Read the model definition and answer for the solid it produces. Units are mm, in the model's axes. A direction names the side the tool comes from. Round coordinates to 2 decimals unless told otherwise and drop trailing zeros. Write each loop counter-clockwise with the first axis right and the second up, starting at its lowest first coordinate (ties: lowest second). Pieces come first, ordered by that corner, then holes. Notation, with made-up numbers: M 21,-13 L 79,-13 A5 cw 79,-7 Z; hole C -14.5,47 d2. An arc over 180 degrees is marked long. Use one line per item in the form item = value. Start each with the question number.
```python
from build123d import *

# Parameters (mm, degrees)
SKETCH1_W               = 101.6
SKETCH1_H               = 6.35
BOSS_EXTRUDE1_DEPTH     = 101.6
CUT_EXTRUDE1_DEPTH      = 144.824345992
SKETCH5_R               = 2.0828
CUT_EXTRUDE2_DEPTH      = 144.824345992
MIRROR2_COPY_1_SKETCH_R = 2.0828
MIRROR2_COPY_1_DEPTH    = 144.824345992


with BuildPart() as part:
    # Sketch1 → Boss-Extrude1 (new body)
    with BuildSketch(Plane(origin=(0, 0, 0), x_dir=(1, 0, 0), z_dir=(0, 1, 0))):
        with Locations((50.8, 3.175)):
            Rectangle(SKETCH1_W, SKETCH1_H)
    extrude(amount=BOSS_EXTRUDE1_DEPTH)

    # Sketch2 → Cut-Extrude1 (cut, through all)
    with BuildSketch(Plane(origin=(0, 0, -6.35), x_dir=(-1, 0, 0), z_dir=(0, 0, -1))):
        with BuildLine():
            Line((-88.9, 66.294), (-12.7, 66.294))
            ThreePointArc((-12.7, 66.294), (-9.906, 63.5), (-12.7, 60.706))
            Line((-12.7, 60.706), (-88.9, 60.706))
            ThreePointArc((-88.9, 60.706), (-91.694, 63.5), (-88.9, 66.294))
        make_face()
        with BuildLine():
            Line((-88.9, 40.894), (-12.7, 40.894))
            ThreePointArc((-12.7, 40.894), (-9.906, 38.1), (-12.7, 35.306))
            Line((-12.7, 35.306), (-88.9, 35.306))
            ThreePointArc((-88.9, 35.306), (-91.694, 38.1), (-88.9, 40.894))
        make_face()
    extrude(amount=-CUT_EXTRUDE1_DEPTH, mode=Mode.SUBTRACT)

    # Sketch5 → Cut-Extrude2 (cut, through all)
    with BuildSketch(Plane.XY):
        with Locations((19.431, 85.725)):
            Circle(SKETCH5_R)
        with Locations((38.481, 95.25)):
            Circle(SKETCH5_R)
        with Locations((38.481, 76.2)):
            Circle(SKETCH5_R)
        with Locations((57.531, 85.725)):
            Circle(SKETCH5_R)
    cut_extrude2 = extrude(amount=-CUT_EXTRUDE2_DEPTH, mode=Mode.SUBTRACT)

    # Mirror1: Cut-Extrude2 across plane
    add(cut_extrude2.mirror(Plane.ZX.offset(50.8)), mode=Mode.SUBTRACT)

    # Mirror2: Cut-Extrude2 across plane
    add(cut_extrude2.mirror(Plane(origin=(48.41875, 0, 0), x_dir=(0, 0, 1), z_dir=(1, 0, 0))), mode=Mode.SUBTRACT)

    # Mirror2 copy 1 sketch → Mirror2 copy 1 (cut, through all)
    with BuildSketch(Plane(origin=(96.8375, 101.6, 0), x_dir=(-1, 0, 0), z_dir=(0, 0, 1))):
        with Locations((19.431, 85.725)):
            Circle(MIRROR2_COPY_1_SKETCH_R)
        with Locations((38.481, 95.25)):
            Circle(MIRROR2_COPY_1_SKETCH_R)
        with Locations((38.481, 76.2)):
            Circle(MIRROR2_COPY_1_SKETCH_R)
        with Locations((57.531, 85.725)):
            Circle(MIRROR2_COPY_1_SKETCH_R)
    extrude(amount=-MIRROR2_COPY_1_DEPTH, mode=Mode.SUBTRACT)


solid = part.part
```
Q1. Find section A-A on y = 6.35. Write down the section's boundary in (x, z).
Q2. Straight lines are drawn through the part: line 1 (X direction, y = 6.35, z = -1.25); line 2 (Y direction, x = 53.5, z = -3); line 3 (X direction, y = 6, z = -1.5). For each, find the intervals that lie inside material, in ascending order. Write a range as [from, to].
Q3. Find section B-B on x = 62. Write down the section's boundary in (y, z).
Q4. For a pull along Y with two mould halves and no side action, classify faces 3 (the face through (50, 0, -3)), 4 (the face through (101.6, 50, -3)), 5 (the face through (91.693, 63.439, -3.219)) as +Y half, -Y half, draft (parallel to the pull), parting line (faces both ways), or undercut.
Q5. A tool of negligible diameter and unlimited length cuts with its end or side. For faces 1 (the face through (50, 50, 0)), 2 (the face through (51, 66.294, -3)), from which of +Z, -Z, +X, -X, +Y, -Y can it reach the whole face along a straight path? Write none if from no direction.
Q6. This flat-tipped pin is pushed along its axis until it touches: pin 1 Ø3.5 at (x, y) = (38.481, 76.2) entering from +Z. Where does it stop, or does it pass through?
Q7. Find section C-C on y = 38.1. Write down the section's boundary in (x, z), and give its area (3 significant figures).
Q8. Find section D-D on z = -1.75. Count the separate pieces of the cut face and the enclosed holes in it, and give its area (3 significant figures).
Response:
q1.outline = M 0,-6.35 L 36.4,-6.35 L 36.4,0 L 0,0 Z; M 40.56,-6.35 L 56.27,-6.35 L 56.27,0 L 40.56,0 Z; M 60.44,-6.35 L 101.6,-6.35 L 101.6,0 L 60.44,0 Z
q2.line_1 = [0, 36.4], [40.56, 56.27], [60.44, 101.6]
q2.line_2 = [0, 35.31], [40.89, 60.71], [66.29, 101.6]
q2.line_3 = [0, 36.43], [40.53, 56.3], [60.41, 101.6]
q3.outline = M 0,-6.35 L 35.31,-6.35 L 35.31,0 L 0,0 Z; M 40.89,-6.35 L 60.71,-6.35 L 60.71,0 L 40.89,0 Z; M 66.29,-6.35 L 101.6,-6.35 L 101.6,0 L 66.29,0 Z
q4.face_3 = -Y half
q4.face_4 = draft
q4.face_5 = undercut
q5.face_1 = +Z, +X, -X, +Y, -Y
q5.face_2 = +Z, -Z
q6.pin_1 = through
q7.outline = M 0,-6.35 L 9.91,-6.35 L 9.91,0 L 0,0 Z; M 91.69,-6.35 L 101.6,-6.35 L 101.6,0 L 91.69,0 Z
q7.area = 126 mm²
q8.separate_pieces = 1
q8.enclosed_holes = 18
q8.area = 9,200 mm²
